For this review, take the finished solid that the model builds, in its own axes (mm). A direction names the side the tool comes from. Round coordinates to 2 decimals unless told otherwise and drop trailing zeros. Write each loop counter-clockwise with the first axis right and the second up, starting at its lowest first coordinate (ties: lowest second). Pieces come first, ordered by that corner, then holes.
Autodesk Inventor part; units mm, degrees
ref_plane "YZ Plane" through (0, 0, 0) normal (1, 0, 0) x (0, 1, 0)
ref_plane "XZ Plane" through (0, 0, 0) normal (0, 1, 0) x (-1, 0, 0)
ref_plane "XY Plane" through (0, 0, 0) normal (0, 0, 1) x (1, 0, 0)
sketch "Sketch1" plane through (0, 0, 0) normal (0, 0, 1) x (1, 0, 0)
  circle A0 centre (-1, 0) radius 36.041 construction
  circle A1 centre (-28.541, 0) radius 8.5 construction
  circle A2 centre (-1, 0) radius 27.541 construction
  circle A3 centre (-1, 27.541) radius 3.3
  circle A4 centre (-1, 0) radius 41.641 construction
  arc A5 (-39.3804, 9.0176) -> (-39.3804, -9.0176) centre (-28.541, 0) ccw
  line L0 (-39.3804, 9.0176) -> (-27.7067, 23.0498)
  line L1 (-39.3804, -9.0176) -> (-27.7067, -23.0498)
  line L2 (0, 0) -> (-50.0981, 0) construction
  arc A6 (-27.7067, -23.0498) -> (-27.7067, 23.0498) centre (0, 0) ccw
  circle A7 centre (-24.8512, 13.7705) radius 3.3
  circle A8 centre (-24.8512, -13.7705) radius 3.3
  circle A9 centre (-1, -27.541) radius 3.3
  circle A10 centre (22.8512, -13.7705) radius 3.3
  circle A11 centre (22.8512, 13.7705) radius 3.3
  line L3 (0, 7.3323) -> (6.35, 3.6662) construction
  line L4 (6.35, 3.6662) -> (6.35, -3.6662) construction
  line L5 (6.35, -3.6662) -> (0, -7.3323) construction
  line L6 (0, -7.3323) -> (-6.35, -3.6662) construction
  line L7 (-6.35, -3.6662) -> (-6.35, 3.6662) construction
  line L8 (-6.35, 3.6662) -> (0, 7.3323) construction
  line L9 (7.55, 4.359) -> (0, 8.718)
  line L10 (0, 8.718) -> (-7.55, 4.359)
  line L11 (-7.55, 4.359) -> (-7.55, -4.359)
  line L12 (-7.55, -4.359) -> (0, -8.718)
  line L13 (0, -8.718) -> (7.55, -4.359)
  line L14 (7.55, -4.359) -> (7.55, 4.359)
  circle A12 centre (-28.541, 0) radius 3.91
  dimension "d2" = 72.082
  dimension "d3" = 17
  dimension "d5" = 6.6
  dimension "d7" = 360
  dimension "d8" = 12.7
  dimension "d9" = 1.2
  dimension "d11" = 7.82
  dimension "d18" = 7.5
  dimension "d19" = 5.6
extrude "Extrusion1" add sketch "Sketch1" along normal blind 3
properties part number "GenevaDrive2" material "Plywood, Finish"
(1) For line 1 along Y through (x, z) = (-1, 1.5); line 2 along Y through (x, z) = (1.5, 2.75); line 3 along X through (y, z) = (14, 0.7), list the stretches that pass through material, from the lowest coordinate up.
Geometry check:
line 1: y = -36.03 to -30.84, -24.24 to -8.14, 8.14 to 24.24, 30.84 to 36.03
line 2: y = -36.01 to -29.7, -25.39 to -7.85, 7.85 to 25.39, 29.7 to 36.01
line 3: x = -35.24 to -28.14, -21.56 to 19.56, 26.14 to 33.21
(2) We need section C-C, the plane y = -28.5. Give the boundary of the cut face in (x, z), and give its area (3 significant figures).
Geometry check:
outline: (-22.06, 0) - (-4.16, 0) - (-4.16, 3) - (-22.06, 3) - close; (2.16, 0) - (22.06, 0) - (22.06, 3) - (2.16, 3) - close
area: 113 mm2
(3) We need section D-D, the plane z = 0.65. State how many separate pieces and enclosed holes the cut face has, and give its area (3 significant figures).
Geometry check:
separate pieces: 1
enclosed holes: 8
area: 3,780 mm2
(4) We need section A-A, the plane y = 0. Give the boundary of the cut face in (x, z), and give its area (3 significant figures).
Geometry check:
outline: (-42.64, 0) - (-32.45, 0) - (-32.45, 3) - (-42.64, 3) - close; (-24.63, 0) - (-7.55, 0) - (-7.55, 3) - (-24.63, 3) - close; (7.55, 0) - (36.04, 0) - (36.04, 3) - (7.55, 3) - close
area: 167 mm2
(5) Mouldability with a two-part tool opening along Y and no side actions: class faces 1 (the face through (-4, 9, 3)), 2 (the face through (36.02, 1.23, 1.48)), 3 (the face through (7.55, 0, 1)) as pulls with the +Y half, pulls with the -Y half, needs draft (parallel to the pull), parting line crosses it, or undercut.
Geometry check:
face 1: needs draft
face 2: parting line crosses it
face 3: undercut
(6) For pin 1 Ø1.5 at (x, z) = (2.5, 0.5) entering from -Y; pin 2 Ø1.5 at (x, z) = (12.5, 1.5) entering from +Y; pin 3 Ø0.9 at (y, z) = (-1.5, 1) entering from +X, all flat-tipped, find the tip position at first contact; note any pin that passes through.
Geometry check:
pin 1: stops at y = -36
pin 2: stops at y = 34.07
pin 3: stops at x = 36.03
(7) We need section B-B, the plane x = -26.5. Give the boundary of the cut face in (y, z), and give its area (3 significant figures).
Geometry check:
outline: (-24.43, 0) - (-16.63, 0) - (-16.63, 3) - (-24.43, 3) - close; (-10.91, 0) - (-3.34, 0) - (-3.34, 3) - (-10.91, 3) - close; (3.34, 0) - (10.91, 0) - (10.91, 3) - (3.34, 3) - close; (16.63, 0) - (24.43, 0) - (24.43, 3) - (16.63, 3) - close
area: 92.3 mm2
(8) For faces 4 (the face through (-33.625, -15.935, 1.479)), 5 (the face through (3.72, -6.57, 1.48)), list the 3-axis set-ups (+Z, -Z, +X, -X, +Y, -Y) from which the entire face can be reached by the end or side of a thin tool; tool diameter is ignored.
Geometry check:
face 4: +Z, -Z, -X, -Y
face 5: +Z, -Z
